```python
from build123d import *

# Parameters (mm, degrees)
F0_R     = 40.5
F0_R_2   = 2.25
F1_DEPTH = 3
F0_R_3   = 43.5
F2_DEPTH = 6


with BuildPart() as f1:
    # F0 (on Top) → F1 (new body)
    with BuildSketch(Plane.XY):
        Circle(F0_R)
        with Locations((-24, -24)):
            Circle(F0_R_2, mode=Mode.SUBTRACT)
        with Locations((-16, -32)):
            Circle(F0_R_2, mode=Mode.SUBTRACT)
        with Locations((-16, -24)):
            Circle(F0_R_2, mode=Mode.SUBTRACT)
        with Locations((-8, -32)):
            Circle(F0_R_2, mode=Mode.SUBTRACT)
        with Locations((-8, -24)):
            Circle(F0_R_2, mode=Mode.SUBTRACT)
        with Locations((-32, -16)):
            Circle(F0_R_2, mode=Mode.SUBTRACT)
        with Locations((-24, -16)):
            Circle(F0_R_2, mode=Mode.SUBTRACT)
        with Locations((-32, -8)):
            Circle(F0_R_2, mode=Mode.SUBTRACT)
        with Locations((-24, -8)):
            Circle(F0_R_2, mode=Mode.SUBTRACT)
        with Locations((-16, -16)):
            Circle(F0_R_2, mode=Mode.SUBTRACT)
        with Locations((-8, -16)):
            Circle(F0_R_2, mode=Mode.SUBTRACT)
        with Locations((-16, -8)):
            Circle(F0_R_2, mode=Mode.SUBTRACT)
        with Locations((-8, -8)):
            Circle(F0_R_2, mode=Mode.SUBTRACT)
        with BuildLine():
            ThreePointArc((0, -34.25), (-2.25, -32), (0, -29.75))
            ThreePointArc((0, -29.75), (1.59099, -30.40901), (2.25, -32))
            ThreePointArc((2.25, -32), (1.59099, -33.59099), (0, -34.25))
        make_face(mode=Mode.SUBTRACT)
        with Locations((8, -32)):
            Circle(F0_R_2, mode=Mode.SUBTRACT)
        with BuildLine():
            ThreePointArc((0, -26.25), (-2.25, -24), (0, -21.75))
            ThreePointArc((0, -21.75), (1.59099, -22.40901), (2.25, -24))
            ThreePointArc((2.25, -24), (1.59099, -25.59099), (0, -26.25))
        make_face(mode=Mode.SUBTRACT)
        with Locations((8, -24)):
            Circle(F0_R_2, mode=Mode.SUBTRACT)
        with Locations((16, -32)):
            Circle(F0_R_2, mode=Mode.SUBTRACT)
        with Locations((16, -24)):
            Circle(F0_R_2, mode=Mode.SUBTRACT)
        with Locations((24, -24)):
            Circle(F0_R_2, mode=Mode.SUBTRACT)
        with BuildLine():
            ThreePointArc((0, -18.25), (-2.25, -16), (0, -13.75))
            ThreePointArc((0, -13.75), (1.59099, -14.40901), (2.25, -16))
            ThreePointArc((2.25, -16), (1.59099, -17.59099), (0, -18.25))
        make_face(mode=Mode.SUBTRACT)
        with Locations((8, -16)):
            Circle(F0_R_2, mode=Mode.SUBTRACT)
        with Locations((16, -16)):
            Circle(F0_R_2, mode=Mode.SUBTRACT)
        with BuildLine():
            ThreePointArc((0, -10.25), (-2.25, -8), (0, -5.75))
            ThreePointArc((0, -5.75), (1.59099, -6.40901), (2.25, -8))
            ThreePointArc((2.25, -8), (1.59099, -9.59099), (0, -10.25))
        make_face(mode=Mode.SUBTRACT)
        with Locations((8, -8)):
            Circle(F0_R_2, mode=Mode.SUBTRACT)
        with Locations((16, -8)):
            Circle(F0_R_2, mode=Mode.SUBTRACT)
        with Locations((24, -16)):
            Circle(F0_R_2, mode=Mode.SUBTRACT)
        with Locations((32, -16)):
            Circle(F0_R_2, mode=Mode.SUBTRACT)
        with Locations((24, -8)):
            Circle(F0_R_2, mode=Mode.SUBTRACT)
        with Locations((32, -8)):
            Circle(F0_R_2, mode=Mode.SUBTRACT)
        with Locations((-32, 0)):
            Circle(F0_R_2, mode=Mode.SUBTRACT)
        with Locations((-24, 0)):
            Circle(F0_R_2, mode=Mode.SUBTRACT)
        with Locations((-32, 8)):
            Circle(F0_R_2, mode=Mode.SUBTRACT)
        with Locations((-24, 8)):
            Circle(F0_R_2, mode=Mode.SUBTRACT)
        with Locations((-32, 16)):
            Circle(F0_R_2, mode=Mode.SUBTRACT)
        with Locations((-24, 16)):
            Circle(F0_R_2, mode=Mode.SUBTRACT)
        with Locations((-16, 0)):
            Circle(F0_R_2, mode=Mode.SUBTRACT)
        with Locations((-16, 8)):
            Circle(F0_R_2, mode=Mode.SUBTRACT)
        with Locations((-8, 0)):
            Circle(F0_R_2, mode=Mode.SUBTRACT)
        with Locations((-8, 8)):
            Circle(F0_R_2, mode=Mode.SUBTRACT)
        with Locations((-16, 16)):
            Circle(F0_R_2, mode=Mode.SUBTRACT)
        with Locations((-8, 16)):
            Circle(F0_R_2, mode=Mode.SUBTRACT)
        with Locations((-24, 24)):
            Circle(F0_R_2, mode=Mode.SUBTRACT)
        with Locations((-16, 24)):
            Circle(F0_R_2, mode=Mode.SUBTRACT)
        with Locations((-16, 32)):
            Circle(F0_R_2, mode=Mode.SUBTRACT)
        with Locations((-8, 24)):
            Circle(F0_R_2, mode=Mode.SUBTRACT)
        with Locations((-8, 32)):
            Circle(F0_R_2, mode=Mode.SUBTRACT)
        with BuildLine():
            ThreePointArc((0, 2.25), (1.59099, 1.59099), (2.25, 0))
            ThreePointArc((2.25, 0), (1.59099, -1.59099), (0, -2.25))
            ThreePointArc((0, -2.25), (-2.25, 0), (0, 2.25))
        make_face(mode=Mode.SUBTRACT)
        with BuildLine():
            ThreePointArc((10.25, 0), (8, -2.25), (5.75, 0))
            ThreePointArc((5.75, 0), (8, 2.25), (10.25, 0))
        make_face(mode=Mode.SUBTRACT)
        with BuildLine():
            ThreePointArc((2.25, 8), (1.59099, 6.40901), (0, 5.75))
            ThreePointArc((0, 5.75), (-2.25, 8), (0, 10.25))
            ThreePointArc((0, 10.25), (1.59099, 9.59099), (2.25, 8))
        make_face(mode=Mode.SUBTRACT)
        with Locations((8, 8)):
            Circle(F0_R_2, mode=Mode.SUBTRACT)
        with BuildLine():
            ThreePointArc((18.25, 0), (16, -2.25), (13.75, 0))
            ThreePointArc((13.75, 0), (16, 2.25), (18.25, 0))
        make_face(mode=Mode.SUBTRACT)
        with Locations((16, 8)):
            Circle(F0_R_2, mode=Mode.SUBTRACT)
        with BuildLine():
            ThreePointArc((2.25, 16), (1.59099, 14.40901), (0, 13.75))
            ThreePointArc((0, 13.75), (-2.25, 16), (0, 18.25))
            ThreePointArc((0, 18.25), (1.59099, 17.59099), (2.25, 16))
        make_face(mode=Mode.SUBTRACT)
        with Locations((8, 16)):
            Circle(F0_R_2, mode=Mode.SUBTRACT)
        with Locations((16, 16)):
            Circle(F0_R_2, mode=Mode.SUBTRACT)
        with BuildLine():
            ThreePointArc((26.25, 0), (24, -2.25), (21.75, 0))
            ThreePointArc((21.75, 0), (24, 2.25), (26.25, 0))
        make_face(mode=Mode.SUBTRACT)
        with BuildLine():
            ThreePointArc((34.25, 0), (32, -2.25), (29.75, 0))
            ThreePointArc((29.75, 0), (32, 2.25), (34.25, 0))
        make_face(mode=Mode.SUBTRACT)
        with Locations((24, 8)):
            Circle(F0_R_2, mode=Mode.SUBTRACT)
        with Locations((32, 8)):
            Circle(F0_R_2, mode=Mode.SUBTRACT)
        with Locations((24, 16)):
            Circle(F0_R_2, mode=Mode.SUBTRACT)
        with Locations((32, 16)):
            Circle(F0_R_2, mode=Mode.SUBTRACT)
        with BuildLine():
            ThreePointArc((2.25, 24), (1.59099, 22.40901), (0, 21.75))
            ThreePointArc((0, 21.75), (-2.25, 24), (0, 26.25))
            ThreePointArc((0, 26.25), (1.59099, 25.59099), (2.25, 24))
        make_face(mode=Mode.SUBTRACT)
        with Locations((8, 24)):
            Circle(F0_R_2, mode=Mode.SUBTRACT)
        with BuildLine():
            ThreePointArc((2.25, 32), (1.59099, 30.40901), (0, 29.75))
            ThreePointArc((0, 29.75), (-2.25, 32), (0, 34.25))
            ThreePointArc((0, 34.25), (1.59099, 33.59099), (2.25, 32))
        make_face(mode=Mode.SUBTRACT)
        with Locations((8, 32)):
            Circle(F0_R_2, mode=Mode.SUBTRACT)
        with Locations((16, 24)):
            Circle(F0_R_2, mode=Mode.SUBTRACT)
        with Locations((16, 32)):
            Circle(F0_R_2, mode=Mode.SUBTRACT)
        with Locations((24, 24)):
            Circle(F0_R_2, mode=Mode.SUBTRACT)
    extrude(amount=F1_DEPTH)

    # F0 (on Top) → F2 (join)
    with BuildSketch(Plane.XY):
        Circle(F0_R_3)
        Circle(F0_R, mode=Mode.SUBTRACT)
    extrude(amount=F2_DEPTH)


solid = f1.part
```
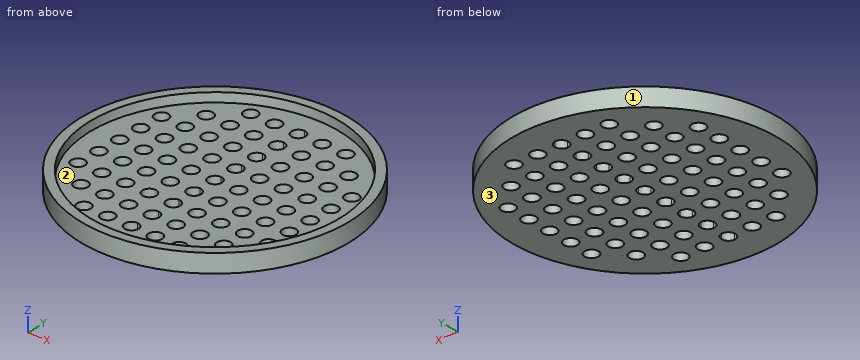
Model file for the job. Use its own axes, mm. Face numbers are marked on the shaded views. Coordinates: 2 decimals unless noted, no trailing zeros. Order: outer loops, then holes, each group sorted by start corner. A loop starts at its lowest first (then second) coordinate and runs counter-clockwise, first axis right, second up. Notation, with made-up numbers: (21, 88) - (72, 88) arc R23 cw to (72, 126) - close; hole circle Ø1 at (69, -23). An arc over 180 degrees is marked (long way). Return JSON: item names as keys, results as strings. Group by question number.
1) Saw through at D-D, the plane y = 38. Write the cut outline in (x, z).
2) Saw through at A-A, the plane x = 32. Write the cut outline in (y, z).
3) Mould opens along Y. For the marked faces 1, 2 and 3 say: released by +Y, released by -Y, zero draft, split by the parting line, or undercut.
4) Saw through at B-B, the plane z = 4.6. Write the cut outline in (x, y), plus the area to 3 significant figures.
5) Saw through at C-C, the plane x = 20. Write the cut outline in (y, z).
6) Probe line 1 (Y direction, x = -33.5, z = 1.25); line 2 (Z direction, x = 6.5, y = 35.5); line 3 (X direction, y = -31, z = 0.85). List the from-to ranges inside material, lowest first. Write a range as from..to.
7) Flat gauge pins, fed straight in: P1, Ø1, axis at x = 24.5, z = 3.5, coming from the -Y side; P2, Ø2, axis at y = 6.5, z = 5, coming from the +X side; P3, Ø6, axis at x = 8, y = 24, coming from the +Z side. Where does each tip first touch, or does it go through?
Values found:
{
 "1": {"outline": "(-21.17, 0) - (21.17, 0) - (21.17, 6) - (14.01, 6) - (14.01, 3) - (-14.01, 3) - (-14.01, 6) - (-21.17, 6) - close"},
 "2": {"outline": "(-29.47, 0) - (-18.25, 0) - (-18.25, 3) - (-24.82, 3) - (-24.82, 6) - (-29.47, 6) - close; (-13.75, 0) - (-10.25, 0) - (-10.25, 3) - (-13.75, 3) - close; (-5.75, 0) - (-2.25, 0) - (-2.25, 3) - (-5.75, 3) - close; (2.25, 0) - (5.75, 0) - (5.75, 3) - (2.25, 3) - close; (10.25, 0) - (13.75, 0) - (13.75, 3) - (10.25, 3) - close; (18.25, 0) - (29.47, 0) - (29.47, 6) - (24.82, 6) - (24.82, 3) - (18.25, 3) - close"},
 "3": {"face 1": "split by the parting line", "face 2": "undercut", "face 3": "zero draft"},
 "4": {"outline": "circle Ø87 at (0, 0); hole circle Ø81 at (0, 0)", "area": "792 mm²"},
 "5": {"outline": "(-38.63, 0) - (38.63, 0) - (38.63, 6) - (35.22, 6) - (35.22, 3) - (-35.22, 3) - (-35.22, 6) - (-38.63, 6) - close"},
 "6": {"line 1": "y = -27.75..-17.68, -14.32..-9.68, -6.32..-1.68, 1.68..6.32, 9.68..14.32, 17.68..27.75", "line 2": "z = 0..3", "line 3": "x = -30.52..-18.02, -13.98..-10.02, -5.98..-2.02, 2.02..5.98, 10.02..13.98, 18.02..30.52"},
 "7": {"P1": "stops at y = -36.28", "P2": "stops at x = 43.15", "P3": "stops at z = 3"}
}
